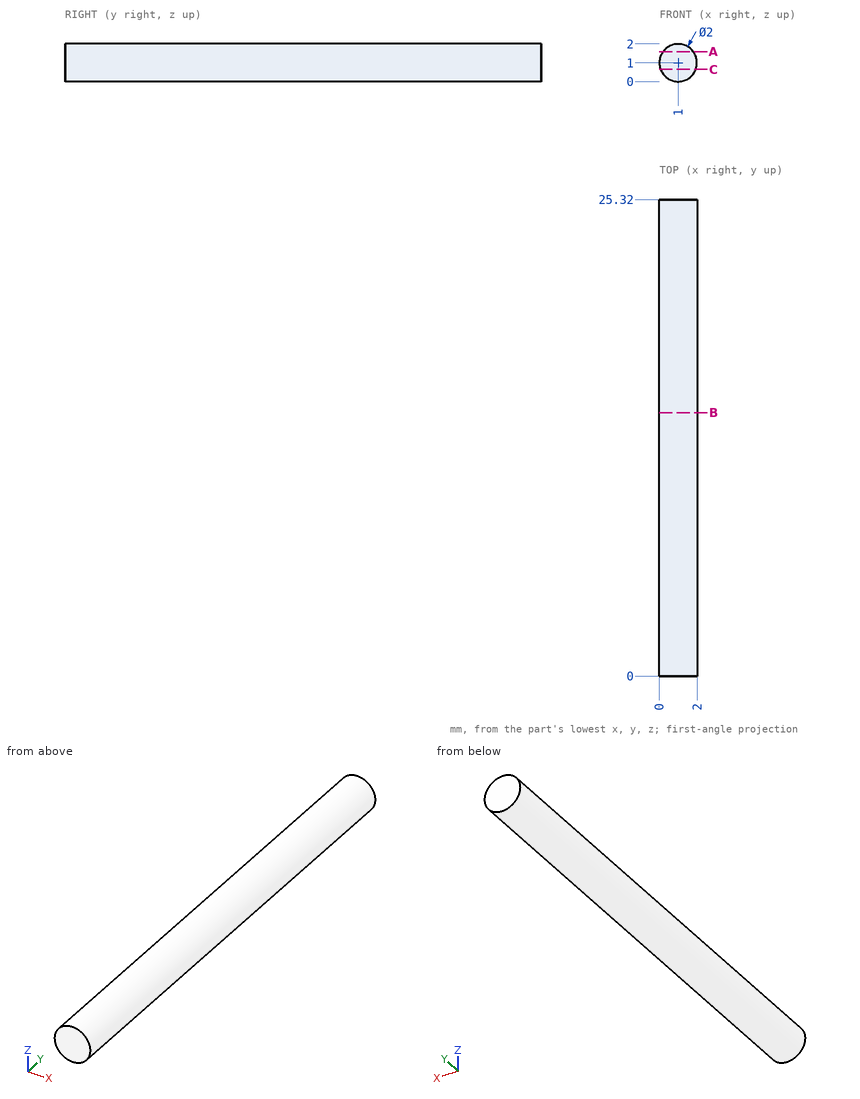
Answer from the drawing. Dimensions are ordinates in mm from the lowest x, y and z of the part. Give positions to 0.01 mm unless a question says otherwise; leave off trailing zeros. Order: outer loops, then holes, each group sorted by start corner. A loop starts at its lowest first (then second) coordinate and runs counter-clockwise, first axis right, second up. Notation, with made-up numbers: (19.5, 13.5) - (77.5, 13.5) arc R18 cw to (77.5, 20.5) - close; hole circle Ø5 at (26, 32.5). An arc over 180 degrees is marked (long way). One line per item, written item: value. Start each with the question number.
1. Section C-C, the plane z = 0.65 is taken. Write down the section's boundary in (x, y).
2. Section A-A, the plane z = 1.6 is taken. Write down the section's boundary in (x, y).
3. Consider line 1 (Z direction, x = 0.95, y = 9); line 2 (Z direction, x = 1.55, y = 6.75); line 3 (X direction, y = 3.75, z = 1.6). Determine where each line is inside the solid, lowest interval first.
4. Section B-B, the plane y = 14 is taken. Write down the section's boundary in (x, z).
Filled sheet:
1. outline: (0.06, 0) - (1.94, 0) - (1.94, 25.32) - (0.06, 25.32) - close
2. outline: (0.2, 0) - (1.8, 0) - (1.8, 25.32) - (0.2, 25.32) - close
3. line 1: 0 to 2
3. line 2: 0.16 to 1.84
3. line 3: 0.2 to 1.8
4. outline: circle Ø2 at (1, 1)
